```python
from build123d import *

# Parameters (mm, degrees)
SKETCH1_R               = 13
BOSS_EXTRUDE1_DEPTH     = 22
SKETCH2_R               = 7
CUT_EXTRUDE1_DEPTH      = 5
SKETCH3_W               = 8.709717948
SKETCH3_H               = 17.861131539
SKETCH3_W_2             = 9.032332804
SKETCH3_H_2             = 17.802474292
CUT_EXTRUDE2_DEPTH      = 14
CUT_EXTRUDE2_DEPTH_BACK = 14
SKETCH4_R               = 2
CUT_EXTRUDE3_DEPTH      = 14
CUT_EXTRUDE3_DEPTH_BACK = 14
CUT_EXTRUDE4_START      = 22
SKETCH5_R               = 3.5
CUT_EXTRUDE4_DEPTH      = 5
SKETCH6_R               = 1.5
CUT_EXTRUDE5_DEPTH      = 23


with BuildPart() as part:
    # Sketch1 → Boss-Extrude1 (new body)
    with BuildSketch(Plane(origin=(0, 0, 0), x_dir=(1, 0, 0), z_dir=(0, 1, 0))):
        Circle(SKETCH1_R)
    extrude(amount=BOSS_EXTRUDE1_DEPTH)

    # Sketch2 → Cut-Extrude1 (cut)
    with BuildSketch(Plane(origin=(0, 0, 0), x_dir=(1, 0, 0), z_dir=(0, 1, 0))):
        Circle(SKETCH2_R)
    extrude(amount=CUT_EXTRUDE1_DEPTH, mode=Mode.SUBTRACT)

    # Sketch3 → Cut-Extrude2 (cut, two sides)
    with BuildSketch(Plane.XY) as cut_extrude2_sk:
        with Locations((9.854858974, 14.93056577)):
            Rectangle(SKETCH3_W, SKETCH3_H)
        with Locations((-10.016166402, 14.901237146)):
            Rectangle(SKETCH3_W_2, SKETCH3_H_2)
    extrude(amount=CUT_EXTRUDE2_DEPTH, mode=Mode.SUBTRACT)
    extrude(cut_extrude2_sk.sketch, amount=-CUT_EXTRUDE2_DEPTH_BACK, mode=Mode.SUBTRACT)

    # Sketch4 → Cut-Extrude3 (cut, two sides)
    with BuildSketch(Plane(origin=(0, 0, 0), x_dir=(0, 0, -1), z_dir=(1, 0, 0))) as cut_extrude3_sk:
        with Locations((-7.5, 13)):
            Circle(SKETCH4_R)
        with Locations((7.5, 13)):
            Circle(SKETCH4_R)
    extrude(amount=CUT_EXTRUDE3_DEPTH, mode=Mode.SUBTRACT)
    extrude(cut_extrude3_sk.sketch, amount=-CUT_EXTRUDE3_DEPTH_BACK, mode=Mode.SUBTRACT)

    # Sketch5 → Cut-Extrude4 (cut)
    with BuildSketch(Plane(origin=(0, 0, 0), x_dir=(1, 0, 0), z_dir=(0, 1, 0)).offset(CUT_EXTRUDE4_START)):
        Circle(SKETCH5_R)
    extrude(amount=-CUT_EXTRUDE4_DEPTH, mode=Mode.SUBTRACT)

    # Sketch6 → Cut-Extrude5 (cut, through all)
    with BuildSketch(Plane(origin=(0, 0, 0), x_dir=(1, 0, 0), z_dir=(0, 1, 0))):
        Circle(SKETCH6_R)
    extrude(amount=CUT_EXTRUDE5_DEPTH, mode=Mode.SUBTRACT)


solid = part.part
```
Geometry: final body of the model. Coordinates: model frame, mm. A direction names the side the tool comes from. Round coordinates to 2 decimals unless told otherwise and drop trailing zeros. Write each loop counter-clockwise with the first axis right and the second up, starting at its lowest first coordinate (ties: lowest second). Pieces come first, ordered by that corner, then holes.
Item 1: Section query D-D (z = 10). Return loops of the section in (x, y), plus the area to 3 significant figures.
Item 2: Mould query, pull axis Z, two halves, no side actions, for faces 5 (the face through (6, 0, 6)), 6 (the face through (0, 5, -2)), 7 (the face through (-1.5, 10.92, -0.07)), 8 (the face through (-12.987, 3.513, -0.572)). Classes: +Z half, -Z half, draft (parallel to the pull), parting line (faces both ways), or undercut.
Item 3: Section query C-C (x = -4.25). Return loops of the section in (y, z).
Item 4: Material intervals for L1, parallel to Z at x = 2.45, y = 13; L2, parallel to Z at x = 0, y = 17.75; L3, parallel to X at y = 18.4, z = 0, sorted ascending.
Item 5: Set-up query: faces 1 (the face through (6.466, 2.465, 2.681)), 2 (the face through (5.5, 14, 0)), 3 (the face through (-8, 6, 0)), 4 (the face through (0, 17, 2)). Return all of +Z, -Z, +X, -X, +Y, -Y with unobstructed straight access to the full face (end or side cutting, diameter ignored); none if empty.
Item 6: Section query B-B (z = 0). Return loops of the section in (x, y), plus the area to 3 significant figures.
Item 7: Pin query (flat end, axial travel): P1, Ø6, axis at x = -10, z = 3.5, coming from the +Y side; P2, Ø2, axis at x = -1.5, z = 1, coming from the +Y side; P3, Ø5, axis at y = 13, z = -7.5, coming from the -X side; P4, Ø6, axis at x = -3, y = 16, coming from the +Z side. Return the tip coordinate at first contact, or that it passes through.
Item 8: Section query A-A (y = 13). Return loops of the section in (x, z), plus the area to 3 significant figures.
Completed:
1. outline: (-8.31, 0) - (8.31, 0) - (8.31, 6) - (5.5, 6) - (5.5, 22) - (-5.5, 22) - (-5.5, 6) - (-8.31, 6) - close
1. area: 276 mm2
2. face 5: draft
2. face 6: undercut
2. face 7: undercut
2. face 8: parting line
3. outline: (0, -12.29) - (22, -12.29) - (22, 12.29) - (0, 12.29) - (0, 5.56) - (5, 5.56) - (5, -5.56) - (0, -5.56) - close; hole circle Ø4 at (13, -7.5); hole circle Ø4 at (13, 7.5)
4. L1: z = -12.77 to -9.5, -5.5 to 5.5, 9.5 to 12.77
4. L2: z = -13 to -3.5, 3.5 to 13
4. L3: x = -5.5 to -3.5, 3.5 to 5.5
5. face 1: -Y
5. face 2: +Z, -Z, +X, +Y
5. face 3: +Z, -Z, -X, +Y
5. face 4: +Y
6. outline: (-13, 0) - (-7, 0) - (-7, 5) - (-1.5, 5) - (-1.5, 17) - (-3.5, 17) - (-3.5, 22) - (-5.5, 22) - (-5.5, 6) - (-13, 6) - close; (1.5, 5) - (7, 5) - (7, 0) - (13, 0) - (13, 6) - (5.5, 6) - (5.5, 22) - (3.5, 22) - (3.5, 17) - (1.5, 17) - close
6. area: 191 mm2
7. P1: stops at y = 6
7. P2: stops at y = 17
7. P3: stops at x = -5.5
7. P4: stops at z = 13
8. outline: (-5.5, -11.78) arc R13 ccw to (5.5, -11.78) - (5.5, -9.5) - (-5.5, -9.5) - close; (-5.5, -5.5) - (5.5, -5.5) - (5.5, 5.5) - (-5.5, 5.5) - close; (-5.5, 9.5) - (5.5, 9.5) - (5.5, 11.78) arc R13 ccw to (-5.5, 11.78) - close; hole circle Ø3 at (0, 0)
8. area: 182 mm2
